from build123d import *
from OCP.BRepFilletAPI import BRepFilletAPI_MakeChamfer

# Parameters (mm, degrees)
BOSS_EXTRUDE1_DEPTH      = 5
BOSS_EXTRUDE2_DEPTH      = 2.5
BOSS_EXTRUDE2_DEPTH_BACK = 2.5
SKETCH6_W                = 5
SKETCH6_H                = 5
SKETCH6_H_2              = 5.343869798
BOSS_EXTRUDE3_DEPTH      = 3
FILLET1_R                = 1
FILLET2_R                = 2
CHAMFER1_SIZE            = 1
CHAMFER1_SIZE2           = 0.363970234
FILLET3_R                = 1


with BuildPart() as part:
    # Sketch1 → Boss-Extrude1 (new body)
    with BuildSketch(Plane.XY):
        Polygon((16.75, 0), (-16.75, 0), (-16.75, 11.5), (-21.75, 11.5), (-21.75, 13.5), (-14.75, 13.5), (-14.75, 2), (14.75, 2), (14.75, 13.5), (21.75, 13.5), (21.75, 11.5), (16.75, 11.5), align=None)
    extrude(amount=-BOSS_EXTRUDE1_DEPTH)

    # Sketch5 → Boss-Extrude2 (add, two sides: drawn at the far end of the back side and taken through both)
    with BuildSketch(Plane(origin=(0, 0, 0), x_dir=(0, 0, -1), z_dir=(1, 0, 0)).offset(-BOSS_EXTRUDE2_DEPTH_BACK)):
        Polygon((19.078065101, 0), (-14.078065101, 0), (-14.078065101, 11.5), (-19.078065101, 11.5), (-19.078065101, 13.5), (-12.078065101, 13.5), (-12.078065101, 2), (17.421934899, 2), (17.421934899, 13.5), (24.421934899, 13.5), (24.421934899, 11.5), (19.078065101, 11.5), align=None)
    extrude(amount=BOSS_EXTRUDE2_DEPTH + BOSS_EXTRUDE2_DEPTH_BACK)

    # Sketch6 → Boss-Extrude3 (add)
    with BuildSketch(Plane(origin=(0, 13.5, 0), x_dir=(1, 0, 0), z_dir=(0, 1, 0))):
        with Locations((19.25, 2.5)):
            Rectangle(SKETCH6_W, SKETCH6_H)
        with Locations((0, -16.578065101)):
            Rectangle(SKETCH6_W, SKETCH6_H)
        with Locations((-19.25, 2.5)):
            Rectangle(SKETCH6_W, SKETCH6_H)
        with Locations((0, 21.75)):
            Rectangle(SKETCH6_W, SKETCH6_H_2)
    extrude(amount=BOSS_EXTRUDE3_DEPTH)

    # Fillet1
    fillet1_edges = [part.edges().sort_by_distance(p)[0] for p in [
        (-14.75, 2, -2.5),
        (14.75, 2, -2.5),
        (0, 2, 12.078065101),
        (0, 2, -17.421934899),
    ]]
    fillet(fillet1_edges, radius=FILLET1_R)

    # Fillet2
    fillet2_edges = [part.edges().sort_by_distance(p)[0] for p in [
        (-21.75, 11.5, -2.5),
        (21.75, 11.5, -2.5),
        (16.75, 0, -2.5),
        (-16.75, 0, -2.5),
        (2.5, 1, 0),
        (-2.5, 1, 0),
        (0, 0, -19.078065101),
        (-2.5, 1, -5),
        (2.5, 1, -5),
        (0, 0, 14.078065101),
        (0, 11.5, 19.078065101),
        (0, 11.5, -24.421934899),
    ]]
    fillet(fillet2_edges, radius=FILLET2_R)

    # Chamfer1: one chamfer whose edges measure the first distance from different faces: ONE call of the kernel's chamfer builder (chamfer() names one face for all edges)
    chamfer1_edges_1 = [part.edges().sort_by_distance(p)[0] for p in [
        (-16.75, 16.5, -2.5),
    ]]
    chamfer1_side_1 = [part.faces().sort_by_distance(p)[0] for p in [
        (-16.75, 15, -2.5),
    ]]
    chamfer1_edges_2 = [part.edges().sort_by_distance(p)[0] for p in [
        (-19.25, 16.5, -5),
    ]]
    chamfer1_side_2 = [part.faces().sort_by_distance(p)[0] for p in [
        (-15.136362203, 7.64232962, -5),
    ]]
    chamfer1_edges_3 = [part.edges().sort_by_distance(p)[0] for p in [
        (-21.75, 16.5, -2.5),
    ]]
    chamfer1_side_3 = [part.faces().sort_by_distance(p)[0] for p in [
        (-21.75, 15, -2.5),
    ]]
    chamfer1_edges_4 = [part.edges().sort_by_distance(p)[0] for p in [
        (-19.25, 16.5, 0),
    ]]
    chamfer1_side_4 = [part.faces().sort_by_distance(p)[0] for p in [
        (-15.136362203, 7.64232962, 0),
    ]]
    chamfer1_edges_5 = [part.edges().sort_by_distance(p)[0] for p in [
        (-2.5, 16.5, -21.75),
    ]]
    chamfer1_side_5 = [part.faces().sort_by_distance(p)[0] for p in [
        (-2.5, 7.829257404, -17.697130979),
    ]]
    chamfer1_edges_6 = [part.edges().sort_by_distance(p)[0] for p in [
        (0, 16.5, -19.078065101),
    ]]
    chamfer1_side_6 = [part.faces().sort_by_distance(p)[0] for p in [
        (0, 15, -19.078065101),
    ]]
    chamfer1_edges_7 = [part.edges().sort_by_distance(p)[0] for p in [
        (2.5, 16.5, -21.75),
    ]]
    chamfer1_side_7 = [part.faces().sort_by_distance(p)[0] for p in [
        (2.5, 7.829257404, -17.697130979),
    ]]
    chamfer1_edges_8 = [part.edges().sort_by_distance(p)[0] for p in [
        (0, 16.5, -24.421934899),
    ]]
    chamfer1_side_8 = [part.faces().sort_by_distance(p)[0] for p in [
        (0, 15, -24.421934899),
    ]]
    chamfer1_edges_9 = [part.edges().sort_by_distance(p)[0] for p in [
        (21.75, 16.5, -2.5),
    ]]
    chamfer1_side_9 = [part.faces().sort_by_distance(p)[0] for p in [
        (21.75, 15, -2.5),
    ]]
    chamfer1_edges_10 = [part.edges().sort_by_distance(p)[0] for p in [
        (19.25, 16.5, -5),
    ]]
    chamfer1_side_10 = [part.faces().sort_by_distance(p)[0] for p in [
        (15.136362203, 7.64232962, -5),
    ]]
    chamfer1_edges_11 = [part.edges().sort_by_distance(p)[0] for p in [
        (16.75, 16.5, -2.5),
    ]]
    chamfer1_side_11 = [part.faces().sort_by_distance(p)[0] for p in [
        (16.75, 15, -2.5),
    ]]
    chamfer1_edges_12 = [part.edges().sort_by_distance(p)[0] for p in [
        (19.25, 16.5, 0),
    ]]
    chamfer1_side_12 = [part.faces().sort_by_distance(p)[0] for p in [
        (15.136362203, 7.64232962, 0),
    ]]
    chamfer1_edges_13 = [part.edges().sort_by_distance(p)[0] for p in [
        (-2.5, 16.5, 16.578065101),
    ]]
    chamfer1_side_13 = [part.faces().sort_by_distance(p)[0] for p in [
        (-2.5, 7.674657573, 12.515775654),
    ]]
    chamfer1_edges_14 = [part.edges().sort_by_distance(p)[0] for p in [
        (0, 16.5, 19.078065101),
    ]]
    chamfer1_side_14 = [part.faces().sort_by_distance(p)[0] for p in [
        (0, 15, 19.078065101),
    ]]
    chamfer1_edges_15 = [part.edges().sort_by_distance(p)[0] for p in [
        (2.5, 16.5, 16.578065101),
    ]]
    chamfer1_side_15 = [part.faces().sort_by_distance(p)[0] for p in [
        (2.5, 7.674657573, 12.515775654),
    ]]
    chamfer1_edges_16 = [part.edges().sort_by_distance(p)[0] for p in [
        (0, 16.5, 14.078065101),
    ]]
    chamfer1_side_16 = [part.faces().sort_by_distance(p)[0] for p in [
        (0, 15, 14.078065101),
    ]]
    chamfer1 = BRepFilletAPI_MakeChamfer(part.part.solid().wrapped)
    for e in chamfer1_edges_1:
        chamfer1.Add(CHAMFER1_SIZE, CHAMFER1_SIZE2, e.wrapped, chamfer1_side_1[0].wrapped)  # the first distance lies on this face
    for e in chamfer1_edges_2:
        chamfer1.Add(CHAMFER1_SIZE, CHAMFER1_SIZE2, e.wrapped, chamfer1_side_2[0].wrapped)  # the first distance lies on this face
    for e in chamfer1_edges_3:
        chamfer1.Add(CHAMFER1_SIZE, CHAMFER1_SIZE2, e.wrapped, chamfer1_side_3[0].wrapped)  # the first distance lies on this face
    for e in chamfer1_edges_4:
        chamfer1.Add(CHAMFER1_SIZE, CHAMFER1_SIZE2, e.wrapped, chamfer1_side_4[0].wrapped)  # the first distance lies on this face
    for e in chamfer1_edges_5:
        chamfer1.Add(CHAMFER1_SIZE, CHAMFER1_SIZE2, e.wrapped, chamfer1_side_5[0].wrapped)  # the first distance lies on this face
    for e in chamfer1_edges_6:
        chamfer1.Add(CHAMFER1_SIZE, CHAMFER1_SIZE2, e.wrapped, chamfer1_side_6[0].wrapped)  # the first distance lies on this face
    for e in chamfer1_edges_7:
        chamfer1.Add(CHAMFER1_SIZE, CHAMFER1_SIZE2, e.wrapped, chamfer1_side_7[0].wrapped)  # the first distance lies on this face
    for e in chamfer1_edges_8:
        chamfer1.Add(CHAMFER1_SIZE, CHAMFER1_SIZE2, e.wrapped, chamfer1_side_8[0].wrapped)  # the first distance lies on this face
    for e in chamfer1_edges_9:
        chamfer1.Add(CHAMFER1_SIZE, CHAMFER1_SIZE2, e.wrapped, chamfer1_side_9[0].wrapped)  # the first distance lies on this face
    for e in chamfer1_edges_10:
        chamfer1.Add(CHAMFER1_SIZE, CHAMFER1_SIZE2, e.wrapped, chamfer1_side_10[0].wrapped)  # the first distance lies on this face
    for e in chamfer1_edges_11:
        chamfer1.Add(CHAMFER1_SIZE, CHAMFER1_SIZE2, e.wrapped, chamfer1_side_11[0].wrapped)  # the first distance lies on this face
    for e in chamfer1_edges_12:
        chamfer1.Add(CHAMFER1_SIZE, CHAMFER1_SIZE2, e.wrapped, chamfer1_side_12[0].wrapped)  # the first distance lies on this face
    for e in chamfer1_edges_13:
        chamfer1.Add(CHAMFER1_SIZE, CHAMFER1_SIZE2, e.wrapped, chamfer1_side_13[0].wrapped)  # the first distance lies on this face
    for e in chamfer1_edges_14:
        chamfer1.Add(CHAMFER1_SIZE, CHAMFER1_SIZE2, e.wrapped, chamfer1_side_14[0].wrapped)  # the first distance lies on this face
    for e in chamfer1_edges_15:
        chamfer1.Add(CHAMFER1_SIZE, CHAMFER1_SIZE2, e.wrapped, chamfer1_side_15[0].wrapped)  # the first distance lies on this face
    for e in chamfer1_edges_16:
        chamfer1.Add(CHAMFER1_SIZE, CHAMFER1_SIZE2, e.wrapped, chamfer1_side_16[0].wrapped)  # the first distance lies on this face
    add(Compound.cast(chamfer1.Shape()), mode=Mode.REPLACE)

    # Fillet3
    fillet3_edges = [part.edges().sort_by_distance(p)[0] for p in [
        (-14.75, 13.5, -2.5),
        (14.75, 13.5, -2.5),
        (0, 13.5, 12.078065101),
        (0, 13.5, -17.421934899),
    ]]
    fillet(fillet3_edges, radius=FILLET3_R)


solid = part.part
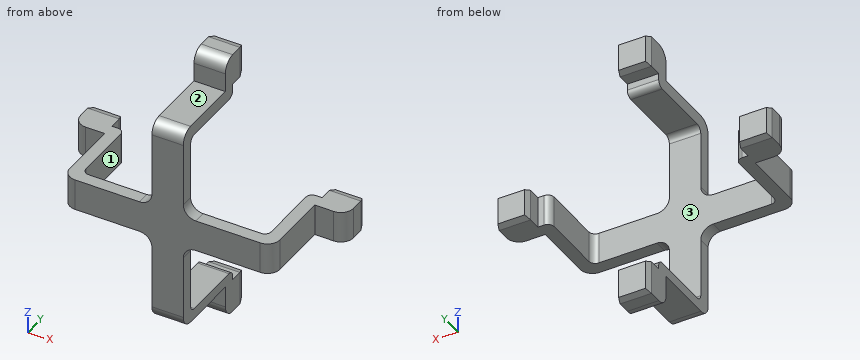
The model under review builds one solid part; all positions refer to its coordinate system, in mm. Face numbers are marked on the shaded views. A direction names the side the tool comes from. Coordinates: 2 decimals unless noted, no trailing zeros. Loops run counter-clockwise (first coordinate to the right, second up) from the corner with the lowest first, then second, coordinate; pieces in that order, holes last. Notation, with made-up numbers: (50, -2) -> (62, -2) arc R25 ccw to (62, 22) -> close; hole circle Ø7 at (32, 3). An arc over 180 degrees is marked (long way). Use a Markdown table: item, result. Add a question column.
1. Add section D-D on x = 11.5. Write out the cut boundary in (y, z).
2. To check wall thickness, follow line 1 (X direction, y = 0.5, z = -12.5); line 2 (Z direction, x = 18.5, y = 12.75); line 3 (X direction, y = 6.25, z = -3.5). State the ranges of each line that lie inside material, in increasing order.
3. Machinability: for the marked faces 1, 2 and 3, which of the approach directions +Z, -Z, +X, -X, +Y, -Y give a long, thin tool a straight path to every point of the face, cutting with its end or side? Answer none if there is none.
4. Add section C-C on z = -1.5. Write out the cut boundary in (x, y).
5. Add section A-A on y = 7.5. Write out the cut boundary in (x, z), plus the area to 3 significant figures.
6. Add section B-B on x = 1.5. Write out the cut boundary in (y, z), plus the area to 3 significant figures.
7. Clearance check with flat-ended pins moving along their axes: pin 1 Ø1.5 at (x, y) = (-2, 6.5) entering from -Z; pin 2 Ø3.5 at (x, z) = (-17.5, -2) entering from -Y; pin 3 Ø8 at (y, z) = (10, 12) entering from -X; pin 4 Ø4 at (x, y) = (6, 5) entering from -Z. State where each tip first meets the part, or that it passes through.
Returned:
| question | item | result |
|---|---|---|
| 1 | outline | (0, -5) -> (2, -5) -> (2, 0) -> (0, 0) -> close |
| 2 | line 1 | x = -2.5 to 2.5 |
| 2 | line 2 | z = -5 to 0 |
| 2 | line 3 | x = -16.75 to -14.75, 14.75 to 16.75 |
| 3 | face 1 | +Z, -Z, +Y |
| 3 | face 2 | +Z, +X, -X, -Y |
| 3 | face 3 | +Y |
| 4 | outline | (-21.75, 13.5) arc R2 ccw to (-19.75, 11.5) -> (-16.75, 11.5) -> (-16.75, 2) arc R2 ccw to (-14.75, 0) -> (14.75, 0) arc R2 ccw to (16.75, 2) -> (16.75, 11.5) -> (19.75, 11.5) arc R2 ccw to (21.75, 13.5) -> (21.75, 15.5) -> (21.39, 16.5) -> (17.11, 16.5) -> (16.75, 15.5) -> (16.75, 13.5) -> (15.75, 13.5) arc R1 ccw to (14.75, 12.5) -> (14.75, 3) arc R1 cw to (13.75, 2) -> (-13.75, 2) arc R1 cw to (-14.75, 3) -> (-14.75, 12.5) arc R1 ccw to (-15.75, 13.5) -> (-16.75, 13.5) -> (-16.75, 15.5) -> (-17.11, 16.5) -> (-21.39, 16.5) -> (-21.75, 15.5) -> close |
| 5 | outline | (-16.75, -5) -> (-14.75, -5) -> (-14.75, 0) -> (-16.75, 0) -> close; (-2.5, -19.08) -> (2.5, -19.08) -> (2.5, -17.42) -> (-2.5, -17.42) -> close; (-2.5, 12.08) -> (2.5, 12.08) -> (2.5, 14.08) -> (-2.5, 14.08) -> close; (14.75, -5) -> (16.75, -5) -> (16.75, 0) -> (14.75, 0) -> close |
| 5 | area | 38.3 mm² |
| 6 | outline | (0, -17.08) arc R2 ccw to (2, -19.08) -> (11.5, -19.08) -> (11.5, -22.42) arc R2 ccw to (13.5, -24.42) -> (15.5, -24.42) -> (16.5, -24.06) -> (16.5, -19.44) -> (15.5, -19.08) -> (13.5, -19.08) -> (13.5, -18.42) arc R1 ccw to (12.5, -17.42) -> (3, -17.42) arc R1 cw to (2, -16.42) -> (2, 11.08) arc R1 cw to (3, 12.08) -> (12.5, 12.08) arc R1 ccw to (13.5, 13.08) -> (13.5, 14.08) -> (15.5, 14.08) -> (16.5, 14.44) -> (16.5, 18.71) -> (15.5, 19.08) -> (13.5, 19.08) arc R2 ccw to (11.5, 17.08) -> (11.5, 14.08) -> (2, 14.08) arc R2 ccw to (0, 12.08) -> close |
| 6 | area | 156 mm² |
| 7 | pin 1 | stops at z = -19.08 |
| 7 | pin 2 | stops at y = 0.27 |
| 7 | pin 3 | stops at x = -2.5 |
| 7 | pin 4 | passes through |
